Input: part model. Units: mm. Frame: model coordinates. A direction names the side the tool comes from. Give positions to 0.01 mm unless a question says otherwise; leave off trailing zeros. Loops run counter-clockwise (first coordinate to the right, second up) from the corner with the lowest first, then second, coordinate; pieces in that order, holes last. Notation, with made-up numbers: (6, 45.25) -> (18, 45.25) arc R22 cw to (18, 65.25) -> close; hole circle Ø7 at (-15, -32.5). An arc over 180 degrees is marked (long way). Use CSV: the item, a comma, the result in double quotes.
Autodesk Inventor part; units mm, degrees
ref_plane "Work Plane1" through (0, 2134.1182, 0) normal (0, 1, 0) x (1, 0, 0)
ref_plane "YZ Plane" through (0, 0, 0) normal (1, 0, 0) x (0, 1, 0)
ref_plane "XZ Plane" through (0, 0, 0) normal (0, 1, 0) x (-1, 0, 0)
sketch "Sketch1" plane through (0, 0, 0) normal (0, 1, 0) x (-1, 0, 0)
  line L0 (0, 0) -> (-615.95, 0)
  line L1 (-615.95, 0) -> (-615.95, -615.95)
  line L2 (-615.95, -615.95) -> (0, -615.95)
  line L3 (0, -615.95) -> (0, 0)
  line L4 (-38.1, -38.1) -> (-577.85, -38.1)
  line L5 (-577.85, -38.1) -> (-577.85, -577.85)
  line L6 (-577.85, -577.85) -> (-38.1, -577.85)
  line L7 (-38.1, -577.85) -> (-38.1, -38.1)
  dimension "d0" = 615.95
  dimension "d2" = 615.95
  dimension "d3" = 38.1
  dimension "d4" = 38.1
  dimension "d5" = 38.1
  dimension "d6" = 38.1
extrude "Extrusion1" add sketch "Sketch1" along normal blind 3.175
sketch "Sketch2" plane through (0, 3.175, 0) normal (0, 1, 0) x (1, 0, 0)
  line L0 (0, 0) -> (615.95, 0)
  line L1 (615.95, 0) -> (615.95, 615.95)
  line L2 (0, 0) -> (615.95, 0)
  line L3 (615.95, 0) -> (615.95, 615.95)
  line L4 (615.95, 615.95) -> (0, 615.95)
  line L5 (0, 615.95) -> (0, 0)
  line L6 (3.175, 3.175) -> (612.775, 3.175)
  line L7 (612.775, 3.175) -> (612.775, 612.775)
  line L8 (612.775, 612.775) -> (3.175, 612.775)
  line L9 (3.175, 612.775) -> (3.175, 3.175)
  dimension "d9" = 3.175
  dimension "d11" = 3.175
  dimension "d12" = 3.175
  dimension "d13" = 3.175
extrude "Extrusion2" add sketch "Sketch2" along normal blind 34.925
sketch "Sketch3" plane through (0, 38.1, 0) normal (0, 1, 0) x (1, 0, 0)
  line L0 (3.175, 3.175) -> (3.175, 612.775)
  line L1 (612.775, 3.175) -> (3.175, 3.175)
  line L2 (0, 0) -> (615.95, 0)
  line L3 (0, 615.95) -> (0, 0)
  line L4 (3.175, 3.175) -> (3.175, 38.1)
  line L5 (0, 38.1) -> (0, 0)
  line L6 (38.1, 0) -> (38.1, 3.175)
  line L7 (0, 38.1) -> (3.175, 38.1)
  dimension "d16" = 38.1
  dimension "d17" = 38.1
  dimension "d18" = 38.1
extrude "Extrusion3" add sketch "Sketch3" along normal blind 2063.75
sketch "Sketch4" plane through (0, 38.1, 0) normal (0, 1, 0) x (1, 0, 0)
  line L0 (612.775, 612.775) -> (612.775, 3.175)
  line L1 (612.775, 3.175) -> (38.1, 3.175)
  line L2 (38.1, 0) -> (615.95, 0)
  line L3 (615.95, 0) -> (615.95, 615.95)
  line L4 (612.775, 3.175) -> (577.85, 3.175)
  line L5 (577.85, 0) -> (615.95, 0)
  line L6 (615.95, 38.1) -> (612.775, 38.1)
  line L7 (577.85, 0) -> (577.85, 3.175)
  point P0 (0, 0)
  dimension "d21" = 38.1
  dimension "d22" = 38.1
  dimension "d23" = 34.925
extrude "Extrusion4" add sketch "Sketch4" along normal blind 2063.75
sketch "Sketch5" plane through (0, 38.1, 0) normal (0, 1, 0) x (1, 0, 0)
  line L0 (615.95, 38.1) -> (615.95, 615.95)
  line L1 (615.95, 615.95) -> (0, 615.95)
  line L2 (3.175, 612.775) -> (612.775, 612.775)
  line L3 (612.775, 612.775) -> (612.775, 38.1)
  line L4 (612.775, 612.775) -> (577.85, 612.775)
  line L5 (577.85, 615.95) -> (615.95, 615.95)
  line L6 (615.95, 577.85) -> (612.775, 577.85)
  line L7 (577.85, 612.775) -> (577.85, 615.95)
  point P0 (0, 0)
  dimension "d26" = 38.1
  dimension "d27" = 38.1
  dimension "d28" = 38.1
extrude "Extrusion5" add sketch "Sketch5" along normal blind 2063.75
sketch "Sketch6" plane through (0, 38.1, 0) normal (0, 1, 0) x (1, 0, 0)
  line L0 (577.85, 615.95) -> (0, 615.95)
  line L1 (0, 615.95) -> (0, 38.1)
  line L2 (3.175, 38.1) -> (3.175, 612.775)
  line L3 (3.175, 612.775) -> (577.85, 612.775)
  line L4 (0, 615.95) -> (0, 577.85)
  line L5 (3.175, 577.85) -> (3.175, 612.775)
  line L6 (38.1, 612.775) -> (38.1, 615.95)
  line L7 (0, 577.85) -> (3.175, 577.85)
  point P0 (0, 0)
  dimension "d31" = 38.1
  dimension "d32" = 38.1
  dimension "d33" = 38.1
extrude "Extrusion6" add sketch "Sketch6" along normal blind 2063.75
sketch "Sketch7" plane through (0, 3.175, 0) normal (0, 1, 0) x (1, 0, 0)
  line L0 (3.175, 612.775) -> (3.175, 3.175)
  line L1 (3.175, 612.775) -> (5.8318, 612.775)
  line L2 (5.8318, 612.775) -> (5.8318, 3.175)
  line L3 (5.8318, 3.175) -> (3.175, 3.175)
  line L4 (3.175, 3.175) -> (3.175, 612.775)
  point P0 (0, 0)
  dimension "d36" = 609.6
  dimension "d38" = 2.6568
extrude "Extrusion7" add sketch "Sketch7" along normal blind 2133.6
sketch "Sketch8" plane through (0, 3.175, 0) normal (0, 1, 0) x (1, 0, 0)
  line L0 (612.775, 3.175) -> (612.775, 612.775)
  line L1 (612.775, 612.775) -> (610.1182, 612.775)
  line L2 (610.1182, 612.775) -> (610.1182, 3.175)
  line L3 (610.1182, 3.175) -> (612.775, 3.175)
  line L4 (612.775, 3.175) -> (612.775, 612.775)
  point P0 (0, 0)
  dimension "d41" = 609.6
  dimension "d43" = 2.6568
extrude "Extrusion8" add sketch "Sketch8" along normal blind 2133.6
sketch "Sketch9" plane through (0, 3.175, 0) normal (0, 1, 0) x (1, 0, 0)
  line L0 (610.1182, 612.775) -> (5.8318, 612.775)
  line L1 (5.8318, 612.775) -> (610.1182, 612.775)
  line L2 (610.1182, 612.775) -> (610.1182, 610.1182)
  line L3 (610.1182, 610.1182) -> (5.8318, 610.1182)
  line L4 (5.8318, 610.1182) -> (5.8318, 612.775)
  point P0 (0, 0)
  dimension "d46" = 604.2863
  dimension "d48" = 2.6568
extrude "Extrusion9" add sketch "Sketch9" along normal blind 2133.6
sketch "Sketch10" plane through (0, 3.175, 0) normal (0, 1, 0) x (1, 0, 0)
  line L0 (5.8318, 3.175) -> (610.1182, 3.175)
  line L1 (5.8318, 3.175) -> (610.1182, 3.175)
  line L2 (610.1182, 3.175) -> (610.1182, 5.8318)
  line L3 (610.1182, 5.8318) -> (5.8318, 5.8318)
  line L4 (5.8318, 5.8318) -> (5.8318, 3.175)
  point P0 (0, 0)
  dimension "d51" = 604.2863
  dimension "d53" = 2.6568
extrude "Extrusion10" add sketch "Sketch10" along normal blind 2133.6
sketch "Sketch11" plane through (0, 2101.85, 0) normal (0, 1, 0) x (1, 0, 0)
  line L0 (577.85, 0) -> (615.95, 0)
  line L1 (612.775, 38.1) -> (612.775, 3.175)
  line L2 (615.95, 0) -> (0, 0)
  line L3 (0, 0) -> (0, 615.95)
  line L4 (0, 615.95) -> (615.95, 615.95)
  line L5 (615.95, 615.95) -> (615.95, 0)
  line L6 (612.775, 3.175) -> (3.175, 3.175)
  line L7 (3.175, 3.175) -> (3.175, 612.775)
  line L8 (3.175, 612.775) -> (612.775, 612.775)
  line L9 (612.775, 612.775) -> (612.775, 3.175)
  point P0 (0, 0)
  dimension "d56" = 615.95
  dimension "d58" = 615.95
  dimension "d59" = 609.6
  dimension "d60" = 609.6
extrude "Extrusion11" add sketch "Sketch11" along normal blind 38.1
sketch "Sketch12" plane through (0, 2136.775, 0) normal (0, 1, 0) x (1, 0, 0)
  line L0 (3.175, 612.775) -> (3.175, 3.175)
  line L1 (3.175, 612.775) -> (612.775, 612.775)
  line L2 (612.775, 612.775) -> (612.775, 3.175)
  line L3 (612.775, 3.175) -> (3.175, 3.175)
  line L4 (3.175, 3.175) -> (3.175, 612.775)
  line L5 (38.1, 577.85) -> (577.85, 577.85)
  line L6 (577.85, 577.85) -> (577.85, 38.1)
  line L7 (577.85, 38.1) -> (38.1, 38.1)
  line L8 (38.1, 38.1) -> (38.1, 577.85)
  line L9 (0, 615.95) -> (0, 0)
  line L10 (615.95, 615.95) -> (0, 615.95)
  dimension "d63" = 609.6
  dimension "d65" = 609.6
  dimension "d66" = 38.1
  dimension "d67" = 38.1
  dimension "d68" = 539.75
  dimension "d69" = 539.75
extrude "Extrusion12" add sketch "Sketch12" along normal blind 3.175
ref_plane "Work Plane1" through (0, 2134.1182, 0) normal (0, 1, 0) x (1, 0, 0)
sketch "Sketch13" plane through (0, 2134.1182, 0) normal (0, 1, 0) x (1, 0, 0)
  line L0 (5.8318, 5.8318) -> (610.1182, 5.8318)
  line L1 (610.1182, 5.8318) -> (610.1182, 610.1182)
  line L2 (610.1182, 610.1182) -> (5.8318, 610.1182)
  line L3 (5.8318, 610.1182) -> (5.8318, 5.8318)
  line L4 (0, 0) -> (615.95, 0)
  line L5 (0, 615.95) -> (0, 0)
  dimension "d73" = 5.8318
  dimension "d74" = 5.8318
  dimension "d75" = 604.2863
  dimension "d76" = 604.2863
extrude "Extrusion13" add sketch "Sketch13" along normal blind 2.6568
sketch "Sketch14" plane through (38.1, 38.1, -3.175) normal (0, 0, 1) x (1, 0, 0)
  line L0 (539.75, 2063.75) -> (0, 2063.75)
  line L1 (0, 0) -> (0, 2063.75)
  line L2 (539.75, 0) -> (0, 0)
  line L3 (539.75, 0) -> (539.75, 2063.75)
  line L4 (63.5, 2000.25) -> (476.25, 2000.25)
  line L5 (476.25, 2000.25) -> (476.25, 1898.65)
  line L6 (476.25, 1898.65) -> (63.5, 1898.65)
  line L7 (63.5, 1898.65) -> (63.5, 2000.25)
  line L8 (63.5, 1797.05) -> (476.25, 1797.05)
  line L9 (476.25, 1797.05) -> (476.25, 266.7)
  line L10 (476.25, 266.7) -> (63.5, 266.7)
  line L11 (63.5, 266.7) -> (63.5, 1797.05)
  line L12 (63.5, 165.1) -> (476.25, 165.1)
  line L13 (476.25, 165.1) -> (476.25, 63.5)
  line L14 (476.25, 63.5) -> (63.5, 63.5)
  line L15 (63.5, 63.5) -> (63.5, 165.1)
  point P0 (-38.1, -38.1)
  dimension "d79" = 63.5
  dimension "d80" = 63.5
  dimension "d81" = 63.5
  dimension "d82" = 101.6
  dimension "d83" = 101.6
  dimension "d84" = 0
  dimension "d85" = 0
  dimension "d86" = 63.5
  dimension "d87" = 101.6
  dimension "d88" = 101.6
  dimension "d89" = 0
  dimension "d90" = 0
extrude "Extrusion14" cut sketch "Sketch14" against normal blind 2.6568 contours L4 L5 L6 L7 | L8 L9 L10 L11 | L12 L13 L14 L15
sketch "Sketch15" plane through (577.85, 38.1, -612.775) normal (0, 0, -1) x (-1, 0, 0)
  line L0 (539.75, 2063.75) -> (0, 2063.75)
  line L1 (0, 0) -> (0, 2063.75)
  line L2 (539.75, 0) -> (0, 0)
  line L3 (539.75, 0) -> (539.75, 2063.75)
  line L4 (63.5, 2000.25) -> (476.25, 2000.25)
  line L5 (476.25, 2000.25) -> (476.25, 1898.65)
  line L6 (476.25, 1898.65) -> (63.5, 1898.65)
  line L7 (63.5, 1898.65) -> (63.5, 2000.25)
  line L8 (63.5, 1797.05) -> (476.25, 1797.05)
  line L9 (476.25, 1797.05) -> (476.25, 266.7)
  line L10 (476.25, 266.7) -> (63.5, 266.7)
  line L11 (63.5, 266.7) -> (63.5, 1797.05)
  line L12 (63.5, 165.1) -> (476.25, 165.1)
  line L13 (476.25, 165.1) -> (476.25, 63.5)
  line L14 (476.25, 63.5) -> (63.5, 63.5)
  line L15 (63.5, 63.5) -> (63.5, 165.1)
  point P0 (577.85, -38.1)
  dimension "d93" = 63.5
  dimension "d94" = 63.5
  dimension "d95" = 63.5
  dimension "d96" = 101.6
  dimension "d97" = 101.6
  dimension "d98" = 0
  dimension "d99" = 0
  dimension "d100" = 101.6
  dimension "d101" = 101.6
  dimension "d102" = 63.5
  dimension "d103" = 0
  dimension "d104" = 0
extrude "Extrusion15" cut sketch "Sketch15" against normal blind 2.6568 contours L4 L5 L6 L7 | L8 L9 L10 L11 | L12 L13 L14 L15
properties part number "Cabinet_2x2x7"
1) Section query B-B (x = 557.5). Return loops of the section in (y, z) (3 decimals), then the cut area to 3 significant figures.
From the geometry:
outline,"(0, -615.95) -> (38.1, -615.95) -> (38.1, -612.775) -> (2101.85, -612.775) -> (2101.85, -615.95) -> (2139.95, -615.95) -> (2139.95, -577.85) -> (2136.775, -577.85) -> (2136.775, -38.1) -> (2139.95, -38.1) -> (2139.95, 0) -> (2101.85, 0) -> (2101.85, -3.175) -> (38.1, -3.175) -> (38.1, 0) -> (0, 0) -> (0, -38.1) -> (3.175, -38.1) -> (3.175, -5.832) -> (2134.118, -5.832) -> (2134.118, -610.118) -> (3.175, -610.118) -> (3.175, -577.85) -> (0, -577.85) -> close"
area,"13,900 mm^2"
2) Ray query, line 1 (Z direction, x = 518, y = 1865.5) (3 decimals); line 2 (X direction, y = 1098, z = -382) (3 decimals); line 3 (Z direction, x = 591.5, y = 893.5). Return the intervals inside material, ascending.
From the geometry:
line 1,"z = -612.775 to -610.118, -5.832 to -3.175"
line 2,"x = 3.175 to 5.832, 610.118 to 612.775"
line 3,"z = -615.95 to -610.12, -5.83 to 0"
3) Reachability of faces 1 (the flat face through (304, 2134.118, -312)), 2 (the flat face through (612.775, 1056, -304)), 3 (the flat face through (87, 989, -3.175)), 4 (the flat face through (3.175, 1056, -312)) from +Z, -Z, +X, -X, +Y, -Y: full face, straight path, thin tool, end or side. Return the list, or none.
From the geometry:
face 1,"none"
face 2,"+X"
face 3,"+Z"
face 4,"-X"
4) Contact query for flat-ended pins moving along their axis: pin 1 (2 mm diameter, centred on x = 367.5, z = -472.5, fed in from +Y) (3 decimals); pin 2 (5 mm diameter, centred on y = 1394, z = -77.5, fed in from -X) (3 decimals); pin 3 (12 mm diameter, centred on x = 410.5, z = -388, fed in from -Y). Output: stop coordinate, or through.
From the geometry:
pin 1,"stops at y = 2136.775"
pin 2,"stops at x = 3.175"
pin 3,"stops at y = 2134.12"
5) Section query C-C (z = -110). Return loops of the section in (x, y) (3 decimals), then the cut area to 3 significant figures.
From the geometry:
outline,"(0, 0) -> (38.1, 0) -> (38.1, 3.175) -> (5.832, 3.175) -> (5.832, 2134.118) -> (610.118, 2134.118) -> (610.118, 3.175) -> (577.85, 3.175) -> (577.85, 0) -> (615.95, 0) -> (615.95, 38.1) -> (612.775, 38.1) -> (612.775, 2101.85) -> (615.95, 2101.85) -> (615.95, 2139.95) -> (577.85, 2139.95) -> (577.85, 2136.775) -> (38.1, 2136.775) -> (38.1, 2139.95) -> (0, 2139.95) -> (0, 2101.85) -> (3.175, 2101.85) -> (3.175, 38.1) -> (0, 38.1) -> close"
area,"13,900 mm^2"
6) Section query D-D (y = 282). Return loops of the section in (x, z) (3 decimals), then the cut area to 3 significant figures.
From the geometry:
outline,"(0, -615.95) -> (38.1, -615.95) -> (38.1, -612.775) -> (577.85, -612.775) -> (577.85, -615.95) -> (615.95, -615.95) -> (615.95, -577.85) -> (612.775, -577.85) -> (612.775, -38.1) -> (615.95, -38.1) -> (615.95, 0) -> (577.85, 0) -> (577.85, -3.175) -> (38.1, -3.175) -> (38.1, 0) -> (0, 0) -> (0, -38.1) -> (3.175, -38.1) -> (3.175, -577.85) -> (0, -577.85) -> close; hole (5.832, -610.118) -> (610.118, -610.118) -> (610.118, -5.832) -> (5.832, -5.832) -> close"
area,"7,380 mm^2"
7) Mould query, pull axis Y, two halves, no side actions, for faces 5 (the flat face through (529, 989, -612.775)), 6 (the flat face through (33, 906, -615.95)), 7 (the flat face through (304, 2136.775, -312)). Classes: pulls with the +Y half, pulls with the -Y half, needs draft (parallel to the pull), parting line crosses it, or undercut.
From the geometry:
face 5,"undercut"
face 6,"needs draft"
face 7,"pulls with the +Y half"
